from build123d import *

# Parameters (mm, degrees)
SKETCH1_R           = 4
SKETCH1_W           = 29
SKETCH1_H           = 6
BOSS_EXTRUDE1_DEPTH = 22
SKETCH2_W           = 8
SKETCH2_H           = 3.96875
CUT_EXTRUDE1_DEPTH  = 33.46921619
BOSS_EXTRUDE2_START = 1
SKETCH3_R           = 4
BOSS_EXTRUDE2_DEPTH = 1
SKETCH4_R           = 1.25
CUT_EXTRUDE2_DEPTH  = 33.56148031
SKETCH5_R           = 1.25
CUT_EXTRUDE3_DEPTH  = 33.46921619
CUT_EXTRUDE4_DEPTH  = 3
SKETCH7_R           = 1
CUT_EXTRUDE5_DEPTH  = 4
SKETCH8_R           = 2.375
CUT_EXTRUDE6_DEPTH  = 1.6


with BuildPart() as part:
    # Sketch1 → Boss-Extrude1 (new body)
    with BuildSketch(Plane.XY):
        with Locations((-18.5, -1)):
            Circle(SKETCH1_R)
        with BuildLine():
            Line((-14.5, -1), (-14.5, 3))
            Line((-14.5, 3), (-18.5, 3))
            ThreePointArc((-18.5, 3), (-15.671572875, 1.828427125), (-14.5, -1))
        make_face()
        with BuildLine():
            Line((-14.5, -3), (-14.5, -1))
            ThreePointArc((-14.5, -1), (-14.636296695, -2.03527618), (-15.035898385, -3))
            Line((-15.035898385, -3), (-14.5, -3))
        make_face()
        Rectangle(SKETCH1_W, SKETCH1_H)
        with BuildLine():
            ThreePointArc((15.035898385, -3), (14.636296695, -2.03527618), (14.5, -1))
            Line((14.5, -1), (14.5, -3))
            Line((14.5, -3), (15.035898385, -3))
        make_face()
        with Locations((18.5, -1)):
            Circle(SKETCH1_R)
        with BuildLine():
            ThreePointArc((14.5, -1), (15.671572875, 1.828427125), (18.5, 3))
            Line((18.5, 3), (14.5, 3))
            Line((14.5, 3), (14.5, -1))
        make_face()
    extrude(amount=BOSS_EXTRUDE1_DEPTH)

    # Sketch2 → Cut-Extrude1 (cut, through all)
    with BuildSketch(Plane(origin=(0, 3, 0), x_dir=(1, 0, 0), z_dir=(0, 1, 0))):
        with Locations((-18.5, -20.015625)):
            Rectangle(SKETCH2_W, SKETCH2_H)
        with Locations((18.5, -20.015625)):
            Rectangle(SKETCH2_W, SKETCH2_H)
    extrude(amount=-CUT_EXTRUDE1_DEPTH, mode=Mode.SUBTRACT)

    # Sketch3 → Boss-Extrude2 (add)
    with BuildSketch(Plane(origin=(0, 0, 0), x_dir=(-1, 0, 0), z_dir=(0, 0, -1)).offset(BOSS_EXTRUDE2_START)):
        with Locations((-18.5, -1)):
            Circle(SKETCH3_R)
        with Locations((18.5, -1)):
            Circle(SKETCH3_R)
    extrude(amount=-BOSS_EXTRUDE2_DEPTH)

    # Sketch4 → Cut-Extrude2 (cut, through all)
    with BuildSketch(Plane(origin=(0, 0, -1), x_dir=(-1, 0, 0), z_dir=(0, 0, -1))):
        with Locations((-18.5, -1)):
            Circle(SKETCH4_R)
        with Locations((18.5, -1)):
            Circle(SKETCH4_R)
    extrude(amount=-CUT_EXTRUDE2_DEPTH, mode=Mode.SUBTRACT)

    # Sketch5 → Cut-Extrude3 (cut, through all)
    with BuildSketch(Plane(origin=(0, 3, 0), x_dir=(1, 0, 0), z_dir=(0, 1, 0))):
        with Locations(Location((-10.75, -5.25, 0), (0, 0, 180))):
            Circle(SKETCH5_R)
        with Locations(Location((10.75, -5.25, 0), (0, 0, 180))):
            Circle(SKETCH5_R)
        with Locations(Location((10.75, -15.75, 0), (0, 0, 180))):
            Circle(SKETCH5_R)
        with Locations(Location((-10.75, -15.75, 0), (0, 0, 180))):
            Circle(SKETCH5_R)
    extrude(amount=-CUT_EXTRUDE3_DEPTH, mode=Mode.SUBTRACT)

    # Sketch6 → Cut-Extrude4 (cut)
    with BuildSketch(Plane.XZ.offset(3)):
        with BuildLine():
            Line((-6.852885683, 2), (6.852885683, 2))
            ThreePointArc((6.852885683, 2), (7.718911087, 2.5), (7.718911087, 3.5))
            ThreePointArc((7.718911087, 3.5), (8.275126266, 7.724873734), (12.5, 8.281088913))
            ThreePointArc((12.5, 8.281088913), (13.5, 8.281088913), (14, 9.147114317))
            Line((14, 9.147114317), (14, 11.852885683))
            ThreePointArc((14, 11.852885683), (13.5, 12.718911087), (12.5, 12.718911087))
            ThreePointArc((12.5, 12.718911087), (9, 12.718911087), (7.25, 15.75))
            Line((7.25, 15.75), (7.25, 22))
            Line((7.25, 22), (-7.25, 22))
            Line((-7.25, 22), (-7.25, 15.75))
            ThreePointArc((-7.25, 15.75), (-9, 12.718911087), (-12.5, 12.718911087))
            ThreePointArc((-12.5, 12.718911087), (-13.5, 12.718911087), (-14, 11.852885683))
            Line((-14, 11.852885683), (-14, 9.147114317))
            ThreePointArc((-14, 9.147114317), (-13.5, 8.281088913), (-12.5, 8.281088913))
            ThreePointArc((-12.5, 8.281088913), (-8.275126266, 7.724873734), (-7.718911087, 3.5))
            ThreePointArc((-7.718911087, 3.5), (-7.718911087, 2.5), (-6.852885683, 2))
        make_face()
    extrude(amount=-CUT_EXTRUDE4_DEPTH, mode=Mode.SUBTRACT)

    # Sketch7 → Cut-Extrude5 (cut)
    with BuildSketch(Plane.XY.offset(22)):
        with Locations((-11.5, -1.5)):
            Circle(SKETCH7_R)
        with Locations((11.5, -1.5)):
            Circle(SKETCH7_R)
    extrude(amount=-CUT_EXTRUDE5_DEPTH, mode=Mode.SUBTRACT)

    # Sketch8 → Cut-Extrude6 (cut)
    with BuildSketch(Plane(origin=(0, 3, 0), x_dir=(1, 0, 0), z_dir=(0, 1, 0))):
        with Locations(Location((-10.75, -5.25, 0), (0, 0, 180))):
            Circle(SKETCH8_R)
        with Locations(Location((10.75, -5.25, 0), (0, 0, 180))):
            Circle(SKETCH8_R)
        with Locations(Location((10.75, -15.75, 0), (0, 0, 180))):
            Circle(SKETCH8_R)
        with Locations(Location((-10.75, -15.75, 0), (0, 0, 180))):
            Circle(SKETCH8_R)
    extrude(amount=-CUT_EXTRUDE6_DEPTH, mode=Mode.SUBTRACT)


solid = part.part
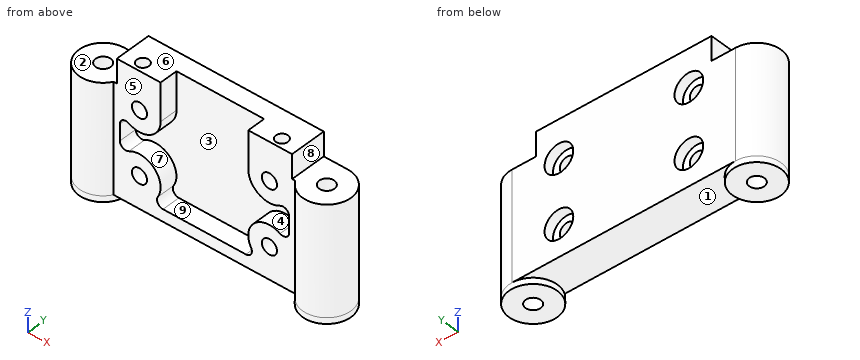
Work out the finished part from the listing and answer in its coordinate system (mm). Face numbers are marked on the shaded views. A direction names the side the tool comes from. Give positions to 0.01 mm unless a question says otherwise; leave off trailing zeros. Write each loop counter-clockwise with the first axis right and the second up, starting at its lowest first coordinate (ties: lowest second). Pieces come first, ordered by that corner, then holes. Notation, with made-up numbers: (69, 50) - (100, 50) arc R15 cw to (100, 73) - close; hole circle Ø1 at (61.5, 23). An arc over 180 degrees is marked (long way). One line per item, written item: value. Start each with the question number.
1. Find section D-D (x = 11.5). Write down the section's boundary in (y, z), then the cut area to 3 significant figures.
2. Consider probe 1 along Z at (x, y) = (-10.75, 2.7) (3 decimals); probe 2 along Z at (x, y) = (-10.75, 0.4); probe 3 along Y at (x, z) = (-11.5, 19.8). Determine where each line is inside the solid, lowest interval first.
3. Find section C-C (y = 2). Write down the section's boundary in (x, z) (3 decimals), then the cut area to 3 significant figures.
4. Find section A-A (z = 5.25). Write down the section's boundary in (x, y) (3 decimals).
5. Given pin 1 (4 mm diameter, centred on x = -10.75, z = 5.25, fed in from +Y); pin 2 (3 mm diameter, centred on x = 6, y = 0.5, fed in from -Z); pin 3 (10 mm diameter, centred on x = -7, z = 4, fed in from -Y); pin 4 (2 mm diameter, centred on x = 10.75, z = 15.75, fed in from +Y), each flat-ended and moving along its own axis, determine where each tip first touches the part or whether it passes through.
6. For a pull along Z with two mould halves and no side action, classify the marked faces 1, 2, 3 and 4 as +Z half, -Z half, draft (parallel to the pull), parting line (faces both ways), or undercut.
7. For the marked faces 5, 6, 7, 8 and 9, determine the directions among +Z, -Z, +X, -X, +Y, -Y from which every point of the face is accessible in a straight line to the end or side of a thin tool.
8. Find section B-B (z = 20.25). Write down the section's boundary in (x, y), then the cut area to 3 significant figures.
Geometry results:
1. outline: (-3, 0) - (3, 0) - (3, 3) - (1.4, 3) - (1.4, 4.25) - (-3, 4.25) - close; (-3, 6.25) - (1.4, 6.25) - (1.4, 7.5) - (3, 7.5) - (3, 13.5) - (1.4, 13.5) - (1.4, 14.75) - (-3, 14.75) - (-3, 12.33) - (0, 12.33) - (0, 8.67) - (-3, 8.67) - close; (-3, 16.75) - (1.4, 16.75) - (1.4, 18) - (3, 18) - (3, 22) - (-0.5, 22) - (-0.5, 18) - (-2.5, 18) - (-2.5, 22) - (-3, 22) - close
1. area: 81.0 mm2
2. probe 1: 0 to 2.875, 7.625 to 13.375, 18.125 to 22
2. probe 2: 0 to 4, 6.5 to 14.5, 17 to 22
2. probe 3: -3 to -2.5, -0.5 to 3
3. outline: (-21.146, -1) - (-15.854, -1) - (-15.854, 0) - (15.854, 0) - (15.854, -1) - (21.146, -1) - (21.146, 18.031) - (14.5, 18.031) - (14.5, 22) - (-14.5, 22) - (-14.5, 18.031) - (-21.146, 18.031) - close; hole circle Ø4.75 at (-10.75, 5.25); hole circle Ø4.75 at (-10.75, 15.75); hole circle Ø4.75 at (10.75, 5.25); hole circle Ø4.75 at (10.75, 15.75)
3. area: 817 mm2
4. outline: (-18.5, 3) arc R4 ccw (long way) to (-15.036, -3) - (-12, -3) - (-12, 1.4) - (-13.125, 1.4) - (-13.125, 3) - close; (-9.5, -3) - (-7.25, -3) - (-7.25, 0) - (7.25, 0) - (7.25, -3) - (9.5, -3) - (9.5, 1.4) - (8.375, 1.4) - (8.375, 3) - (-8.375, 3) - (-8.375, 1.4) - (-9.5, 1.4) - close; (12, -3) - (15.036, -3) arc R4 ccw (long way) to (18.5, 3) - (13.125, 3) - (13.125, 1.4) - (12, 1.4) - close; hole circle Ø2.5 at (-18.5, -1); hole circle Ø2.5 at (18.5, -1)
5. pin 1: y = 1.4
5. pin 2: z = 0
5. pin 3: y = -3
5. pin 4: through
6. face 1: -Z half
6. face 2: +Z half
6. face 3: undercut
6. face 4: undercut
7. face 5: +Z, -Z, -Y
7. face 6: +Z, +X, -X, +Y, -Y
7. face 7: -Y
7. face 8: +Z, +X, +Y, -Y
7. face 9: +Z, -Y
8. outline: (-14.5, -3) - (-7.25, -3) - (-7.25, 0) - (7.25, 0) - (7.25, -3) - (14.5, -3) - (14.5, 3) - (-14.5, 3) - close; hole circle Ø2 at (-11.5, -1.5); hole circle Ø2 at (11.5, -1.5)
8. area: 124 mm2
